For this review, take the finished solid that the model builds, in its own axes (mm). A direction names the side the tool comes from. Give positions to 0.01 mm unless a question says otherwise; leave off trailing zeros. Loops run counter-clockwise (first coordinate to the right, second up) from the corner with the lowest first, then second, coordinate; pieces in that order, holes last.
```python
from build123d import *

# Parameters (mm, degrees)
BOSS_EXTRUDE1_DEPTH            = 120
CBORE_FOR_M4_SHCS4_D           = 4.5
CBORE_FOR_M4_SHCS4_CBORE_D     = 8
CBORE_FOR_M4_SHCS4_CBORE_DEPTH = 4
M4_TAPPED_HOLE1_D              = 3.3
M5_TAPPED_HOLE1_D              = 4.2
M5_TAPPED_HOLE1_DEPTH          = 17.4
M5_TAPPED_HOLE1_TIP            = 1.2618073
M4_TAPPED_HOLE2_D              = 3.3
M3_TAPPED_HOLE2_D              = 2.5
M3_TAPPED_HOLE2_DEPTH          = 11.5
M3_TAPPED_HOLE2_TIP            = 0.751075774


with BuildPart() as part:
    # Sketch1 → Boss-Extrude1 (new body)
    with BuildSketch(Plane.XY):
        Polygon((0, 0), (0, 200), (28, 200), (28, 164.5), (14, 164.5), (14, 110.5), (28, 110.5), (28, 0), align=None)
    extrude(amount=BOSS_EXTRUDE1_DEPTH)

    # CBORE for M4 SHCS4 (through all)
    with Locations(Plane(origin=(0, 194, 73), x_dir=(0, 0, -1), z_dir=(-1, 0, 0))):
        with Locations((0, 0), (0, 26), (1, 36.3), (1, 76.3), (0, 86.6), (0, 112.6), (26, 112.6), (26, 86.6), (25, 76.3), (25, 36.3), (26, 26), (26, 0)):
            CounterBoreHole(CBORE_FOR_M4_SHCS4_D / 2, CBORE_FOR_M4_SHCS4_CBORE_D / 2, CBORE_FOR_M4_SHCS4_CBORE_DEPTH)

    # M4 Tapped Hole1 (through all)
    with Locations(Plane(origin=(0, 190, 16.7), x_dir=(0, 0, -1), z_dir=(-1, 0, 0))):
        with Locations((0, 0), (0, 60), (0, 120), (0, 180), (-86.6, 180), (-86.6, 120), (-86.6, 60), (-86.6, 0)):
            Hole(M4_TAPPED_HOLE1_D / 2)

    # M5 Tapped Hole1
    with Locations(Plane(origin=(14, 0, 90), x_dir=(-1, 0, 0), z_dir=(0, -1, 0))):
        with Locations((0, 0), (0, 30), (0, 60)):
            Hole(M5_TAPPED_HOLE1_D / 2, depth=M5_TAPPED_HOLE1_DEPTH)
            with Locations((0, 0, -(M5_TAPPED_HOLE1_DEPTH + M5_TAPPED_HOLE1_TIP / 2))):  # 118° drill point
                Cone(0, M5_TAPPED_HOLE1_D / 2, M5_TAPPED_HOLE1_TIP, mode=Mode.SUBTRACT)

    # M4 Tapped Hole2 (through all)
    with Locations(Plane(origin=(28, 15, 80.1), x_dir=(0, 1, 0), z_dir=(1, 0, 0))):
        with Locations((0, 0), (0, -40)):
            Hole(M4_TAPPED_HOLE2_D / 2)

    # M3 Tapped Hole2
    with Locations(Plane(origin=(28, 103.660435599, 106.9), x_dir=(0, 1, 0), z_dir=(1, 0, 0))):
        with Locations((0, 0), (-22.2, 10.3), (0, -93.8), (-22.2, -104.1)):
            Hole(M3_TAPPED_HOLE2_D / 2, depth=M3_TAPPED_HOLE2_DEPTH)
            with Locations((0, 0, -(M3_TAPPED_HOLE2_DEPTH + M3_TAPPED_HOLE2_TIP / 2))):  # 118° drill point
                Cone(0, M3_TAPPED_HOLE2_D / 2, M3_TAPPED_HOLE2_TIP, mode=Mode.SUBTRACT)


solid = part.part
```
Q1. For pin 1 Ø2 at (y, z) = (70, 16.7) entering from -X; pin 2 Ø4 at (y, z) = (117, 48) entering from -X; pin 3 Ø2 at (y, z) = (81.46, 2.8) entering from +X; pin 4 Ø7 at (y, z) = (117.7, 72) entering from +X, all flat-tipped, find the tip position at first contact; note any pin that passes through.
Answers:
pin 1: passes through
pin 2: stops at x = 4
pin 3: stops at x = 16.35
pin 4: stops at x = 14
Q2. Consider section A-A on x = 19.5. Count the separate pieces of the cut face and the enclosed holes in it, plus the area to 3 significant figures.
Answers:
separate pieces: 2
enclosed holes: 20
area: 17,300 mm2
Q3. Machinability: for faces 4 (the cylindrical face through (16.17, 82.26, 75.08)), 5 (the flat face through (4, 159.4, 70.3)), 6 (the cylindrical face through (13.54, 8.82, 62.05)), which of the approach directions +Z, -Z, +X, -X, +Y, -Y give a long, thin tool a straight path to every point of the face, cutting with its end or side? Answer none if there is none.
Answers:
face 4: +X, -X
face 5: -X
face 6: -Y
Q4. For probe 1 along Z at (x, y) = (19.5, 107.4); probe 2 along Z at (x, y) = (0.8, 194); probe 3 along Y at (x, z) = (23.25, 117.2), list the stretches that pass through material, from the lowest coordinate up.
Answers:
probe 1: z = 0 to 44.75, 49.25 to 70.75, 75.25 to 120
probe 2: z = 0 to 43, 51 to 69, 77 to 120
probe 3: y = 0 to 80.21, 82.71 to 110.5, 164.5 to 200
Q5. Consider section B-B on y = 107.4. Give the boundary of the cut face in (x, z).
Answers:
outline: (0, 0) - (28, 0) - (28, 44.75) - (4, 44.75) - (4, 43) - (0, 43) - close; (0, 51) - (4, 51) - (4, 49.25) - (28, 49.25) - (28, 70.75) - (4, 70.75) - (4, 69) - (0, 69) - close; (0, 77) - (4, 77) - (4, 75.25) - (28, 75.25) - (28, 120) - (0, 120) - close
Q6. Consider section C-C on z = 98.5. Give the boundary of the cut face in (x, y), plus the area to 3 significant figures.
Answers:
outline: (0, 0) - (28, 0) - (28, 110.5) - (14, 110.5) - (14, 164.5) - (28, 164.5) - (28, 200) - (0, 200) - close
area: 4,840 mm2
Q7. Mouldability with a two-part tool opening along Y and no side actions: class faces 1 (the flat face through (28, 182, 59)), 2 (the cylindrical face through (16.168, 195.996, 74.038)), 3 (the conical face through (13.66, 18.44, 30.14)) as +Y half, -Y half, draft (parallel to the pull), parting line (faces both ways), or undercut.
Answers:
face 1: draft
face 2: undercut
face 3: -Y half
